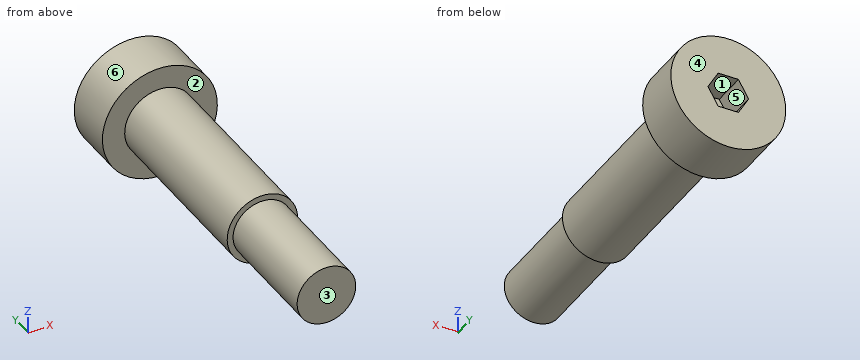
```python
from build123d import *

# Parameters (mm, degrees)
CUT_EXTRUDE_1_DEPTH = 3


with BuildPart() as part:
    # 草图1 → 旋转1 (revolve)
    with BuildSketch(Plane.XY, mode=Mode.PRIVATE) as revolve_1_sk:
        Polygon((0, 0), (0, 30.4), (4.9, 30.4), (4.9, 26), (3, 26), (3, 10), (2.5, 10), (2.5, 0), align=None)
    revolve(revolve_1_sk.sketch.rotate(Axis((0, 0, 0), (0, 1, 0)), 90), axis=Axis((0, 0, 0), (0, 1, 0)))

    # 草图2 → 切除-拉伸1 (cut)
    with BuildSketch(Plane(origin=(0, 30.4, 0), x_dir=(1, 0, 0), z_dir=(0, 1, 0))):
        Polygon((1.732050808, 0), (0.866025404, 1.5), (-0.866025404, 1.5), (-1.732050808, 0), (-0.866025404, -1.5), (0.866025404, -1.5), align=None)
    extrude(amount=-CUT_EXTRUDE_1_DEPTH, mode=Mode.SUBTRACT)


solid = part.part
```
For this review, take the finished solid that the model builds, in its own axes (mm). Face numbers are marked on the shaded views. A direction names the side the tool comes from. Coordinates: 2 decimals unless noted, no trailing zeros. Loops run counter-clockwise (first coordinate to the right, second up) from the corner with the lowest first, then second, coordinate; pieces in that order, holes last. Notation, with made-up numbers: (13, 63.25) - (46, 63.25) arc R24 ccw to (46, 74.25) - close; hole circle Ø9 at (46, 60.25). An arc over 180 degrees is marked (long way). Use one line per item in the form item = value. Start each with the question number.
1) Take a section at C-C (y = 19). State the section outline as (x, z) points.
2) For pin 1 (2.5 mm diameter, centred on x = 0, z = 0, fed in from +Y); pin 2 (4 mm diameter, centred on x = 0.5, y = 4.5, fed in from +Z); pin 3 (2 mm diameter, centred on y = 19, z = -2, fed in from +X); pin 4 (5 mm diameter, centred on x = 2, z = -3, fed in from -Y), all flat-tipped, find the tip position at first contact; note any pin that passes through.
3) Take a section at D-D (x = 3.5). State the section outline as (y, z) points.
4) To check wall thickness, follow probe 1 along Y at (x, z) = (0.5, -3); probe 2 along Y at (x, z) = (0.5, 1.25); probe 3 along Z at (x, y) = (1.5, 28). State the ranges of each line that lie inside material, in increasing order. Write a range as from..to.
5) For the marked faces 1, 2 and 3, list the 3-axis set-ups (+Z, -Z, +X, -X, +Y, -Y) from which the entire face can be reached by the end or side of a thin tool; tool diameter is ignored.
6) Take a section at B-B (z = -1). State the section outline as (x, y) points, plus the area to 3 significant figures.
7) Take a section at A-A (x = 0). State the section outline as (y, z) points, plus the area to 3 significant figures.
8) Draft analysis for pull direction Z (two halves, no side actions). For the marked faces 4, 5 and 6, state which applies: released by +Z, released by -Z, zero draft, split by the parting line, or undercut.
From the geometry:
q1.outline = circle Ø6 at (0, 0)
q2.pin_1 = 27.4
q2.pin_2 = 2.5
q2.pin_3 = 2.83
q2.pin_4 = 0
q3.outline = (26, -3.43) - (30.4, -3.43) - (30.4, 3.43) - (26, 3.43) - close
q4.probe_1 = 26..30.4
q4.probe_2 = 0..27.4
q4.probe_3 = -4.66..-0.4, 0.4..4.66
q5.face_1 = +Y
q5.face_2 = -Y
q5.face_3 = +Z, -Z, +X, -X, -Y
q6.outline = (-4.8, 26) - (-2.83, 26) - (-2.83, 10) - (-2.29, 10) - (-2.29, 0) - (2.29, 0) - (2.29, 10) - (2.83, 10) - (2.83, 26) - (4.8, 26) - (4.8, 30.4) - (1.15, 30.4) - (1.15, 27.4) - (-1.15, 27.4) - (-1.15, 30.4) - (-4.8, 30.4) - close
q6.area = 172 mm2
q7.outline = (0, -2.5) - (10, -2.5) - (10, -3) - (26, -3) - (26, -4.9) - (30.4, -4.9) - (30.4, -1.5) - (27.4, -1.5) - (27.4, 1.5) - (30.4, 1.5) - (30.4, 4.9) - (26, 4.9) - (26, 3) - (10, 3) - (10, 2.5) - (0, 2.5) - close
q7.area = 180 mm2
q8.face_4 = zero draft
q8.face_5 = undercut
q8.face_6 = split by the parting line
